```python
from build123d import *

# Parameters (mm, degrees)
F0_W      = 20
F0_H      = 8
F1_DEPTH  = 5
F2_W      = 20
F2_H      = 0.5
F3_DEPTH  = 10
F5_DEPTH  = 0.5
F7_DEPTH  = 0.5
F8_DEPTH  = 5
F11_W     = 19
F11_H     = 0.5570442975
F12_DEPTH = 4
F14_DEPTH = 25
F15_W     = 19
F15_H     = 9
F16_DEPTH = 7


# Not quite as in the source:
# - a feature of the source that left no trace in its solid (it failed there, or was rolled back) is left out


with BuildPart() as f1:
    # F0 (on Top) → F1 (new body)
    with BuildSketch(Plane.XY):
        with Locations((8.2929818355, 4)):
            Rectangle(F0_W, F0_H)
    extrude(amount=F1_DEPTH)

    # F2 (on face) → F3 (join)
    with BuildSketch(Plane.XY.offset(5)):
        with Locations((8.2929818355, 7.75)):
            Rectangle(F2_W, F2_H)
    extrude(amount=F3_DEPTH)

    # F4 (on face) → F5 (join)
    with BuildSketch(Plane(origin=(-1.7070181645, 0, 0), x_dir=(0, -1, 0), z_dir=(-1, 0, 0))):
        Polygon((-7.5, 5), (0, 5), (-7.5, 15), align=None)
    extrude(amount=-F5_DEPTH)

    # F6 (on face) → F7 (join)
    with BuildSketch(Plane.YZ.offset(18.2929818355)):
        Polygon((7.5, 5), (7.5, 15), (0, 5), align=None)
    extrude(amount=-F7_DEPTH)

    # F8 (add): a face of the model
    f8_faces = [f1.faces().sort_by_distance(p)[0] for p in [
        (8.2929818355, 4, 0),
    ]]
    extrude(f8_faces, amount=F8_DEPTH)

    # F11 (on face) → F12 (join)
    with BuildSketch(Plane.XZ.offset(-7.5)):
        with Locations((8.2929818355, 10.2785221487)):
            Rectangle(F11_W, F11_H)
    extrude(amount=F12_DEPTH)

    # F13 (on face) → F14 (cut)
    with BuildSketch(Plane.YZ.offset(17.7929818355)):
        Polygon((3.75, 10), (4.1247227065, 10.4996302754), (4.1677832231, 10.5570442975), (3.5, 10.5570442975), (3.5, 10), align=None)
    extrude(amount=-F14_DEPTH, mode=Mode.SUBTRACT)

    # F15 (on face) → F16 (cut)
    with BuildSketch(Plane.XZ):
        with Locations((8.2929818355, 0)):
            Rectangle(F15_W, F15_H)
    extrude(amount=-F16_DEPTH, mode=Mode.SUBTRACT)


solid = f1.part
```
Geometry: final body of the model. Coordinates: model frame, mm. A direction names the side the tool comes from. Round coordinates to 2 decimals unless told otherwise and drop trailing zeros. Write each loop counter-clockwise with the first axis right and the second up, starting at its lowest first coordinate (ties: lowest second). Pieces come first, ordered by that corner, then holes. Notation, with made-up numbers: (64, 2.25) -> (115, 2.25) arc R24 ccw to (115, 14.25) -> close; hole circle Ø4 at (7.25, 54.5). An arc over 180 degrees is marked (long way). Return JSON: item names as keys, results as strings.
Q1. Ray query, line 1 (Z direction, x = 4.25, y = 5.75); line 2 (X direction, y = 7.25, z = 7.75); line 3 (Z direction, x = 12.75, y = 7.25). Return the intervals inside material, ascending.
From the geometry:
{"line 1": "-5 to -4.5, 4.5 to 5, 10 to 10.56", "line 2": "-1.71 to -1.21, 17.79 to 18.29", "line 3": "-5 to 5, 10 to 10.56"}
Q2. Set-up query: faces 1 (the flat face through (8, 7.5, 7)), 2 (the flat face through (18.293, 4, 3)), 3 (the flat face through (8, 6, 10.557)). Return all of +Z, -Z, +X, -X, +Y, -Y with unobstructed straight access to the full face (end or side cutting, diameter ignored); none if empty.
From the geometry:
{"face 1": "-Y", "face 2": "+Z, -Z, +X, +Y, -Y", "face 3": "+Z, -Y"}
Q3. First-contact query: pin 1 Ø1.7 at (x, y) = (10.5, 6) entering from +Z; pin 2 Ø12 at (x, z) = (11, 4) entering from -Y; pin 3 Ø2.5 at (x, z) = (7, 7.5) entering from -Y; pin 4 Ø1 at (x, y) = (16, 1) entering from +Z. Flat tips, straight axial feed; report the tip coordinate or a pass-through.
From the geometry:
{"pin 1": "z = 10.56", "pin 2": "y = 0", "pin 3": "y = 7.5", "pin 4": "z = 5"}
Q4. Section A-A on y = 1.5. Return the cut outline in (x, z), and give its area (3 significant figures).
From the geometry:
{"outline": "(-1.71, -5) -> (18.29, -5) -> (18.29, 7) -> (17.79, 7) -> (17.79, 5) -> (-1.21, 5) -> (-1.21, 7) -> (-1.71, 7) -> close; hole (-1.21, -4.5) -> (17.79, -4.5) -> (17.79, 4.5) -> (-1.21, 4.5) -> close", "area": "31.0 mm2"}
Q5. Section C-C on y = 5.25. Return the cut outline in (x, z).
From the geometry:
{"outline": "(-1.71, -5) -> (18.29, -5) -> (18.29, 12) -> (17.79, 12) -> (17.79, 10.56) -> (-1.21, 10.56) -> (-1.21, 12) -> (-1.71, 12) -> close; hole (-1.21, -4.5) -> (17.79, -4.5) -> (17.79, 4.5) -> (-1.21, 4.5) -> close; hole (-1.21, 5) -> (17.79, 5) -> (17.79, 10) -> (-1.21, 10) -> close"}
Q6. Section D-D on z = 2.5. Return the cut outline in (x, y).
From the geometry:
{"outline": "(-1.71, 0) -> (-1.21, 0) -> (-1.21, 7) -> (17.79, 7) -> (17.79, 0) -> (18.29, 0) -> (18.29, 8) -> (-1.71, 8) -> close"}
Q7. Section B-B on x = 12.25. Return the cut outline in (y, z).
From the geometry:
{"outline": "(0, -5) -> (8, -5) -> (8, 15) -> (7.5, 15) -> (7.5, 10.56) -> (4.17, 10.56) -> (3.75, 10) -> (7.5, 10) -> (7.5, 5) -> (0, 5) -> (0, 4.5) -> (7, 4.5) -> (7, -4.5) -> (0, -4.5) -> close"}
